Autodesk Inventor part; units mm, degrees
ref_plane "YZ Plane" through (0, 0, 0) normal (1, 0, 0) x (0, 1, 0)
ref_plane "XZ Plane" through (0, 0, 0) normal (0, 1, 0) x (-1, 0, 0)
ref_plane "XY Plane" through (0, 0, 0) normal (0, 0, 1) x (1, 0, 0)
sketch "Sketch1" plane through (0, 0, 0) normal (0, 0, 1) x (1, 0, 0)
  line L0 (85.72, 30.226) -> (85.72, 1.401) construction
  line L1 (85.72, 1.401) -> (45.72, 1.401) construction
  line L2 (85.72, 1.401) -> (5.72, 1.401) construction
  line L3 (5.72, 1.401) -> (5.72, 59.001) construction
  line L4 (5.72, 59.001) -> (85.72, 59.001) construction
  line L5 (85.72, 59.001) -> (85.72, 1.401) construction
  line L6 (61.99, 1.401) -> (61.99, 20.221) construction
  line L7 (61.99, 20.221) -> (85.72, 20.221) construction
  line L8 (61.99, 20.221) -> (58.44, 20.221) construction
  line L9 (61.99, 23.771) -> (61.99, 20.221) construction
  line L10 (60.215, 20.221) -> (61.99, 20.221) construction
  line L11 (61.99, 20.221) -> (61.99, 21.996) construction
  line L12 (61.99, 21.996) -> (60.215, 21.996) construction
  line L13 (60.215, 21.996) -> (60.215, 20.221) construction
  circle A0 centre (60.215, 21.996) radius 1.775 construction
  circle A1 centre (60.215, 21.996) radius 2.775 construction
  circle A2 centre (60.215, 21.996) radius 4.275 construction
  line L14 (5.72, 59.001) -> (74.72, 59.001) construction
  line L15 (74.72, 59.001) -> (74.72, 53.301) construction
  line L16 (74.72, 53.301) -> (5.72, 53.301) construction
  line L17 (5.72, 53.301) -> (5.72, 59.001) construction
  line L18 (5.72, 1.401) -> (18.72, 1.401) construction
  line L19 (18.72, 1.401) -> (18.72, 14.401) construction
  line L20 (18.72, 14.401) -> (5.72, 14.401) construction
  line L21 (5.72, 14.401) -> (5.72, 1.401) construction
  circle A3 centre (2.72, 58.001) radius 1.5
  line L22 (3.72, 61.001) -> (5.72, 61.001)
  line L23 (5.72, 61.001) -> (5.72, 59.001) construction
  line L24 (5.72, 61.001) -> (2.72, 61.001)
  line L25 (5.72, 55.001) -> (5.72, 61.001) construction
  line L26 (45.72, 1.9437) -> (45.72, 30.226) construction
  line L27 (45.72, 30.226) -> (85.72, 30.226) construction
  arc A4 (2.72, 61.001) -> (1.52, 55.2515) centre (2.72, 58.001) ccw
  circle A5 centre (2.72, 2.451) radius 1.5
  line L28 (3.72, -0.549) -> (5.72, -0.549)
  line L29 (5.72, -0.549) -> (2.72, -0.549)
  arc A6 (1.52, 5.2005) -> (2.72, -0.549) centre (2.72, 2.451) ccw
  circle A7 centre (88.72, 58.001) radius 1.5
  line L30 (85.72, 61.001) -> (88.72, 61.001)
  arc A8 (89.92, 55.2515) -> (88.72, 61.001) centre (88.72, 58.001) ccw
  line L31 (85.72, -0.549) -> (88.72, -0.549)
  circle A9 centre (88.72, 2.451) radius 1.5
  arc A10 (88.72, -0.549) -> (89.92, 5.2005) centre (88.72, 2.451) ccw
  line L32 (2.72, 53.4184) -> (2.72, 7.0336)
  line L33 (5.72, 61.001) -> (85.72, 61.001)
  line L34 (88.72, 53.4184) -> (88.72, 7.0336)
  line L35 (85.72, -0.549) -> (5.72, -0.549)
  arc A11 (2.72, 53.4184) -> (1.52, 55.2515) centre (0.72, 53.4184) ccw
  arc A12 (1.52, 5.2005) -> (2.72, 7.0336) centre (0.72, 7.0336) ccw
  arc A13 (88.72, 7.0336) -> (89.92, 5.2005) centre (90.72, 7.0336) ccw
  arc A14 (89.92, 55.2515) -> (88.72, 53.4184) centre (90.72, 53.4184) ccw
  point P0 (0, 0)
  point P1 (2.72, 55.001)
  point P2 (2.72, 5.451)
  point P3 (91.44, 0)
  point P4 (88.72, 55.001)
  point P5 (88.72, 5.451)
  dimension "d32" = 40
  dimension "d33" = 28.825
  dimension "d34" = 80
  dimension "d37" = 18.82
  dimension "d40" = 5.55
  dimension "d41" = 8.55
  dimension "d42" = 69
  dimension "d43" = 5.7
  dimension "d44" = 13
  dimension "d45" = 13
  dimension "d52" = 2
  dimension "d80" = 3
extrude "Extrusion1" add sketch "Sketch1" along normal blind 2
sketch "Sketch2" plane through (0, 0, 2) normal (0, 0, 1) x (1, 0, 0)
  line L0 (85.72, 30.226) -> (85.72, 1.401)
  line L1 (5.72, 14.401) -> (5.72, 53.301)
  line L2 (74.72, 59.001) -> (85.72, 59.001)
  line L3 (85.72, 59.001) -> (85.72, 1.401)
  line L4 (61.815, 21.996) -> (60.215, 21.996)
  circle A0 centre (60.215, 21.996) radius 1.6
  circle A1 centre (60.215, 21.996) radius 2.775 construction
  circle A2 centre (60.215, 21.996) radius 4.275
  line L5 (45.72, 59.001) -> (74.72, 59.001)
  line L6 (74.72, 59.001) -> (74.72, 53.301)
  line L7 (74.72, 53.301) -> (5.72, 53.301)
  line L8 (5.72, 58.001) -> (5.72, 59.001)
  line L9 (5.72, 1.401) -> (18.72, 1.401)
  line L10 (18.72, 1.401) -> (18.72, 14.401)
  line L11 (18.72, 14.401) -> (5.72, 14.401)
  line L12 (5.72, 2.451) -> (5.72, 1.401)
  circle A3 centre (2.72, 58.001) radius 1.5
  line L13 (3.72, 61.001) -> (5.72, 61.001)
  line L14 (5.72, 61.001) -> (5.72, 59.001)
  line L15 (5.72, 61.001) -> (2.72, 61.001)
  line L16 (5.72, 59.001) -> (5.72, 61.001)
  arc A4 (2.72, 61.001) -> (1.52, 55.2515) centre (2.72, 58.001) ccw
  line L17 (3.72, -0.549) -> (5.72, -0.549)
  line L18 (5.72, -0.549) -> (2.72, -0.549)
  circle A5 centre (2.72, 2.451) radius 1.5
  arc A6 (1.52, 5.2005) -> (2.72, -0.549) centre (2.72, 2.451) ccw
  line L19 (85.72, -0.549) -> (88.72, -0.549)
  circle A7 centre (88.72, 2.451) radius 1.5
  arc A8 (88.72, -0.549) -> (89.92, 5.2005) centre (88.72, 2.451) ccw
  circle A9 centre (88.72, 58.001) radius 1.5
  arc A10 (89.92, 55.2515) -> (88.72, 61.001) centre (88.72, 58.001) ccw
  line L20 (85.72, 61.001) -> (88.72, 61.001)
  line L21 (2.72, 53.4184) -> (2.72, 7.0336)
  line L22 (5.72, 61.001) -> (85.72, 61.001)
  line L23 (88.72, 53.4184) -> (88.72, 7.0336)
  line L24 (85.72, -0.549) -> (5.72, -0.549)
  arc A11 (2.72, 53.4184) -> (1.52, 55.2515) centre (0.72, 53.4184) ccw
  arc A12 (1.52, 5.2005) -> (2.72, 7.0336) centre (0.72, 7.0336) ccw
  arc A13 (88.72, 7.0336) -> (89.92, 5.2005) centre (90.72, 7.0336) ccw
  arc A14 (89.92, 55.2515) -> (88.72, 53.4184) centre (90.72, 53.4184) ccw
  line L25 (85.72, 1.401) -> (74.72, 1.401)
  line L26 (61.99, 1.401) -> (45.72, 1.401)
  line L27 (85.72, 1.401) -> (74.72, 1.401)
  line L28 (61.99, 1.401) -> (18.72, 1.401)
  line L29 (61.99, 1.401) -> (74.72, 1.401)
  point P0 (0, 0)
  point P1 (2.72, 55.001)
  point P2 (2.72, 5.451)
  point P3 (91.44, 0)
  point P4 (88.72, 5.451)
  point P5 (88.72, 55.001)
  dimension "d89" = 3.2
  dimension "d53" = 40
  dimension "d54" = 28.825
  dimension "d55" = 80
  dimension "d57" = 5.55
  dimension "d58" = 8.55
  dimension "d59" = 69
  dimension "d60" = 5.7
  dimension "d61" = 13
  dimension "d62" = 13
  dimension "d63" = 2
  dimension "d81" = 3
  dimension "d82" = 3
  dimension "d83" = 3
  dimension "d84" = 3
extrude "Extrusion2" add sketch "Sketch2" along normal blind 3
sketch "Sketch5" plane through (0, 0, 5) normal (0, 0, 1) x (1, 0, 0)
  line L0 (85.72, 30.226) -> (85.72, 1.401)
  line L1 (85.72, 1.401) -> (45.72, 1.401)
  line L2 (85.72, 1.401) -> (5.72, 1.401)
  line L3 (5.72, 1.401) -> (5.72, 59.001)
  line L4 (5.72, 59.001) -> (85.72, 59.001)
  line L5 (85.72, 59.001) -> (85.72, 1.401)
  line L6 (5.72, 59.001) -> (74.72, 59.001)
  line L7 (5.72, 53.301) -> (5.72, 59.001)
  line L8 (5.72, 1.401) -> (18.72, 1.401)
  line L9 (5.72, 14.401) -> (5.72, 1.401)
  circle A0 centre (2.72, 58.001) radius 1.5
  line L10 (3.72, 61.001) -> (5.72, 61.001)
  line L11 (5.72, 61.001) -> (5.72, 59.001)
  line L12 (5.72, 61.001) -> (2.72, 61.001)
  line L13 (5.72, 55.001) -> (5.72, 61.001)
  arc A1 (2.72, 61.001) -> (1.52, 55.2515) centre (2.72, 58.001) ccw
  line L14 (3.72, -0.549) -> (5.72, -0.549)
  line L15 (5.72, -0.549) -> (2.72, -0.549)
  circle A2 centre (2.72, 2.451) radius 1.5
  arc A3 (1.52, 5.2005) -> (2.72, -0.549) centre (2.72, 2.451) ccw
  line L16 (85.72, -0.549) -> (88.72, -0.549)
  circle A4 centre (88.72, 2.451) radius 1.5
  arc A5 (88.72, -0.549) -> (89.92, 5.2005) centre (88.72, 2.451) ccw
  circle A6 centre (88.72, 58.001) radius 1.5
  arc A7 (89.92, 55.2515) -> (88.72, 61.001) centre (88.72, 58.001) ccw
  line L17 (85.72, 61.001) -> (88.72, 61.001)
  line L18 (2.72, 53.4184) -> (2.72, 7.0336)
  line L19 (5.72, 61.001) -> (85.72, 61.001)
  line L20 (88.72, 53.4184) -> (88.72, 7.0336)
  line L21 (85.72, -0.549) -> (5.72, -0.549)
  arc A8 (2.72, 53.4184) -> (1.52, 55.2515) centre (0.72, 53.4184) ccw
  arc A9 (1.52, 5.2005) -> (2.72, 7.0336) centre (0.72, 7.0336) ccw
  arc A10 (88.72, 7.0336) -> (89.92, 5.2005) centre (90.72, 7.0336) ccw
  arc A11 (89.92, 55.2515) -> (88.72, 53.4184) centre (90.72, 53.4184) ccw
  point P0 (0, 0)
  point P1 (0, 0)
  point P2 (2.72, 55.001)
  point P3 (2.72, 5.451)
  point P4 (91.44, 0)
  point P5 (88.72, 5.451)
  point P6 (88.72, 55.001)
  dimension "d64" = 40
  dimension "d65" = 28.825
  dimension "d66" = 80
  dimension "d74" = 2
  dimension "d85" = 3
  dimension "d86" = 3
  dimension "d87" = 3
  dimension "d88" = 3
extrude "Extrusion5" add sketch "Sketch5" along normal blind 1.67
chamfer "Chamfer1" distance 1 distance2 3 1 edges at (55.94, 21.996, 5) measured on face at (63.5414, 21.5273, 5)
properties part number "Redid Enclosure Bottom"
The model under review builds one solid part; all positions refer to its coordinate system, in mm. A direction names the side the tool comes from. Coordinates: 2 decimals unless noted, no trailing zeros. Write each loop counter-clockwise with the first axis right and the second up, starting at its lowest first coordinate (ties: lowest second). Pieces come first, ordered by that corner, then holes. Notation, with made-up numbers: M 43,36 L 48,36 A12 ccw 48,51 Z; hole C 83.25,61.5 d8. An arc over 180 degrees is marked long. Put each result on its own line as item: value.
1) For faces 4 (the cylindrical face through (89.06, 5.92, 3.29)), 5 (the flat face through (12, 14.401, 3)), 6 (the cylindrical face through (-0.204, 1.782, 3.288)), list the 3-axis set-ups (+Z, -Z, +X, -X, +Y, -Y) from which the entire face can be reached by the end or side of a thin tool; tool diameter is ignored.
Computed:
face 4: +Z, -Z, +X
face 5: +Z
face 6: +Z, -Z, -X
2) Add section C-C on y = 40.5. Give the boundary of the cut face in (x, z).
Computed:
outline: M 2.72,0 L 88.72,0 L 88.72,6.67 L 85.72,6.67 L 85.72,2 L 5.72,2 L 5.72,6.67 L 2.72,6.67 Z
3) Draft analysis for pull direction X (two halves, no side actions). For faces 1 (the cylindrical face through (90.106, 58.576, 3.288)), 2 (the cylindrical face through (89.04, 54.5, 3.29)), 3 (the cylindrical face through (2.4, 5.95, 3.29)), state which applies: released by +X, released by -X, zero draft, split by the parting line, or undercut.
Computed:
face 1: undercut
face 2: released by +X
face 3: released by -X
4) Clearance check with flat-ended pins moving along their axes: pin 1 Ø4.5 at (x, y) = (37, 56.5) entering from +Z; pin 2 Ø1.5 at (y, z) = (9.5, 4) entering from +X; pin 3 Ø0.9 at (y, z) = (56.5, 4) entering from +X. State where each tip first meets the part, or that it passes through.
Computed:
pin 1: stops at z = 5
pin 2: stops at x = 88.72
pin 3: stops at x = 91.53
5) Add section A-A on z = 3.75. Give the boundary of the cut face in (x, y) (1 decimal).
Computed:
outline: M 1.5,5.2 A3 ccw 2.7,-0.5 L 88.7,-0.5 A3 ccw 89.9,5.2 A2 cw 88.7,7 L 88.7,53.4 A2 cw 89.9,55.3 A3 ccw 88.7,61 L 2.7,61 A3 ccw 1.5,55.3 A2 cw 2.7,53.4 L 2.7,7 A2 cw Z; C 60.2,22 d7.4; hole C 2.7,2.5 d3; hole C 2.7,58 d3; hole M 5.7,14.4 L 18.7,14.4 L 18.7,1.4 L 85.7,1.4 L 85.7,59 L 74.7,59 L 74.7,53.3 L 5.7,53.3 Z; hole C 60.2,22 d3.2; hole C 88.7,2.5 d3; hole C 88.7,58 d3
6) Add section B-B on x = 28. Give the boundary of the cut face in (y, z), then the cut area to 3 significant figures.
Computed:
outline: M -0.55,0 L 61,0 L 61,6.67 L 59,6.67 L 59,5 L 53.3,5 L 53.3,2 L 1.4,2 L 1.4,6.67 L -0.55,6.67 Z
area: 159 mm2
7) Add section D-D on x = 11. Give the boundary of the cut face in (y, z).
Computed:
outline: M -0.55,0 L 61,0 L 61,6.67 L 59,6.67 L 59,5 L 53.3,5 L 53.3,2 L 14.4,2 L 14.4,5 L 1.4,5 L 1.4,6.67 L -0.55,6.67 Z
8) Wall thickness on probe 1 along Y at (x, z) = (50, 6.5); probe 2 along X at (y, z) = (7, 6); probe 3 along X at (y, z) = (58, 4.5): over which ranges is each line inside the solid? List them lowest first. Write a range as [from, to].
Computed:
probe 1: y = [-0.55, 1.4], [59, 61]
probe 2: x = [2.72, 5.72], [85.72, 88.72]
probe 3: x = [-0.28, 1.22], [4.22, 74.72], [85.72, 87.22], [90.22, 91.72]
